```python
from build123d import *

# Parameters (mm, degrees)
SKETCH1_R           = 3.175
BOSS_EXTRUDE1_DEPTH = 1.5875
SKETCH2_R           = 20.6375
BOSS_EXTRUDE2_DEPTH = 25.4
FILLET1_R           = 9.525


with BuildPart() as part:
    # Sketch1 → Boss-Extrude1 (new body)
    with BuildSketch(Plane(origin=(0, 0, 0), x_dir=(1, 0, 0), z_dir=(0, 1, 0))):
        with BuildLine():
            ThreePointArc((-18.941091873, 16.316710411), (-25, 0), (-18.941091873, -16.316710411))
            Line((-18.941091873, -16.316710411), (-4.811037336, -32.719444444))
            ThreePointArc((-4.811037336, -32.719444444), (0, -34.925), (4.811037336, -32.719444444))
            Line((4.811037336, -32.719444444), (18.941091873, -16.316710411))
            ThreePointArc((18.941091873, -16.316710411), (25, 0), (18.941091873, 16.316710411))
            Line((18.941091873, 16.316710411), (4.811037336, 32.719444444))
            ThreePointArc((4.811037336, 32.719444444), (0, 34.925), (-4.811037336, 32.719444444))
            Line((-4.811037336, 32.719444444), (-18.941091873, 16.316710411))
        make_face()
        with Locations(Location((0, -28.575, 0), (0, 0, 270))):
            Circle(SKETCH1_R, mode=Mode.SUBTRACT)
        with Locations(Location((0, 28.575, 0), (0, 0, 270))):
            Circle(SKETCH1_R, mode=Mode.SUBTRACT)
    extrude(amount=BOSS_EXTRUDE1_DEPTH)

    # Sketch2 → Boss-Extrude2 (add)
    with BuildSketch(Plane(origin=(0, 1.5875, 0), x_dir=(1, 0, 0), z_dir=(0, 1, 0))):
        with Locations(Location((0, 0, 0), (0, 0, 270))):
            Circle(SKETCH2_R)
    extrude(amount=BOSS_EXTRUDE2_DEPTH)

    # Fillet1
    fillet1_edges = [part.edges().sort_by_distance(p)[0] for p in [
        (0, 26.9875, -20.6375),
    ]]
    fillet(fillet1_edges, radius=FILLET1_R)

    # Sketch4 → Revolve1 (revolve)
    with BuildSketch(Plane(origin=(0, 0, 0), x_dir=(0, 0, -1), z_dir=(1, 0, 0))):
        with BuildLine():
            Line((10.998522628, 26.9875), (0, 26.9875))
            Line((0, 26.9875), (0, 33.3375))
            ThreePointArc((0, 33.3375), (6.35, 31.636022628), (10.998522628, 26.9875))
        make_face()
    revolve(axis=Axis((0, 26.9875, 0), (0, 1, 0)))


solid = part.part
```
Read the model definition and answer for the solid it produces. Units are mm, in the model's axes. A direction names the side the tool comes from. Give positions to 0.01 mm unless a question says otherwise; leave off trailing zeros. Order: outer loops, then holes, each group sorted by start corner. A loop starts at its lowest first (then second) coordinate and runs counter-clockwise, first axis right, second up.
(1) For a pull along Z with two mould halves and no side action, classify faces 3 (the cylindrical face through (-1.932, 0.783, -31.095)), 4 (the cylindrical face through (-1.932, 0.783, 26.055)), 5 (the cylindrical face through (25, 1, 0)), 6 (the flat face through (0, 1.588, -21)) as released by +Z, released by -Z, zero draft, split by the parting line, or undercut.
(2) Find section D-D (y = 12.5). Give the vertices of the cut face in (x, z) (1 decimal).
(3) Find section B-B (x = 0). Give the number of separate pieces and of enclosed holes in the cut face, plus the area to 3 significant figures.
(4) Find section A-A (z = -26.5). Give the vertices of the cut face in (x, y).
(5) For faces 1 (the cylindrical face through (20.46, 9.41, -2.69)), 2 (the flat face through (-11.78, 0.78, -24.63)), determine the directions among +Z, -Z, +X, -X, +Y, -Y from which every point of the face is accessible in a straight line to the end or side of a thin tool.
(6) Given pin 1 (4 mm diameter, centred on x = -4, z = -7.5, fed in from -Y); pin 2 (3 mm diameter, centred on x = -13, z = 6, fed in from +Y); pin 3 (25 mm diameter, centred on x = 12, z = -8.5, fed in from +Y); pin 4 (3 mm diameter, centred on y = 26.5, z = -3, fed in from +X), each flat-ended and moving along its own axis, determine where each tip first touches the part or whether it passes through.
(7) Straight lines are drawn through the part: L1, parallel to Y at x = 11.5, z = 19.5; L2, parallel to Y at x = 4, z = -10.5; L3, parallel to X at y = 2.5, z = -5. For each, find the intervals that lie inside material, in ascending order.
Result sheet:
1. face 3: undercut
1. face 4: undercut
1. face 5: split by the parting line
1. face 6: zero draft
2. outline: circle Ø41.3 at (0, 0)
3. separate pieces: 3
3. enclosed holes: 0
3. area: 1,200 mm2
4. outline: (-10.17, 0) - (-2.4, 0) - (-2.4, 1.59) - (-10.17, 1.59) - close; (2.4, 0) - (10.17, 0) - (10.17, 1.59) - (2.4, 1.59) - close
5. face 1: +Y
5. face 2: -Z, -X, +Y, -Y
6. pin 1: stops at y = 0
6. pin 2: stops at y = 26.83
6. pin 3: stops at y = 33.14
6. pin 4: stops at x = 16.69
7. L1: y = 0 to 1.59
7. L2: y = 0 to 26.99
7. L3: x = -20.02 to 20.02
